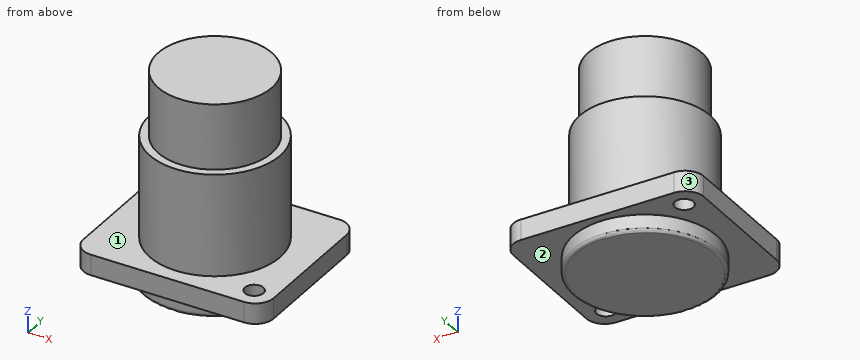
from build123d import *

# Parameters (mm, degrees)
SZKIC1_R                    = 11.6
DODANIE_WYCI_GNI_CIE1_DEPTH = 2.7
ZAOKR_GLENIE1_R             = 0.5
SZKIC2_W                    = 30.8
SZKIC2_H                    = 25.8
DODANIE_WYCI_GNI_CIE2_DEPTH = 3.33
SZKIC3_R                    = 10.55
DODANIE_WYCI_GNI_CIE3_DEPTH = 16.5
SZKIC4_R                    = 9.2
DODANIE_WYCI_GNI_CIE4_DEPTH = 10.6
SZKIC5_R                    = 1.5
WYTNIJ_WYCI_GNI_CIE1_DEPTH  = 10.6
ZAOKR_GLENIE2_R             = 3


with BuildPart() as part:
    # Szkic1 → Dodanie-wyciągnięcie1 (new body)
    with BuildSketch(Plane.XY):
        with Locations(Location((0, 0, 0), (0, 0, 180))):
            Circle(SZKIC1_R)
    extrude(amount=DODANIE_WYCI_GNI_CIE1_DEPTH)

    # Zaokrąglenie1
    zaokr_glenie1_edges = [part.edges().sort_by_distance(p)[0] for p in [
        (11.6, 0, 0),
    ]]
    fillet(zaokr_glenie1_edges, radius=ZAOKR_GLENIE1_R)

    # Szkic2 → Dodanie-wyciągnięcie2 (add)
    with BuildSketch(Plane.XY.offset(2.7)):
        Rectangle(SZKIC2_W, SZKIC2_H)
    extrude(amount=DODANIE_WYCI_GNI_CIE2_DEPTH)

    # Szkic3 → Dodanie-wyciągnięcie3 (add)
    with BuildSketch(Plane.XY.offset(6.03)):
        Circle(SZKIC3_R)
    extrude(amount=DODANIE_WYCI_GNI_CIE3_DEPTH)

    # Szkic4 → Dodanie-wyciągnięcie4 (add)
    with BuildSketch(Plane.XY.offset(22.53)):
        Circle(SZKIC4_R)
    extrude(amount=DODANIE_WYCI_GNI_CIE4_DEPTH)

    # Szkic5 → Wytnij-wyciągnięcie1 (cut)
    with BuildSketch(Plane(origin=(0, 0, 2.7), x_dir=(-1, 0, 0), z_dir=(0, 0, -1))):
        with Locations((-12, -9.5)):
            Circle(SZKIC5_R)
        with Locations((12, 9.5)):
            Circle(SZKIC5_R)
    extrude(amount=-WYTNIJ_WYCI_GNI_CIE1_DEPTH, mode=Mode.SUBTRACT)

    # Zaokrąglenie2
    zaokr_glenie2_edges = [part.edges().sort_by_distance(p)[0] for p in [
        (-15.4, 12.9, 4.365),
        (-15.4, -12.9, 4.365),
        (15.4, -12.9, 4.365),
        (15.4, 12.9, 4.365),
    ]]
    fillet(zaokr_glenie2_edges, radius=ZAOKR_GLENIE2_R)


solid = part.part
Read the model definition and answer for the solid it produces. Units are mm, in the model's axes. Face numbers are marked on the shaded views. A direction names the side the tool comes from. Coordinates: 2 decimals unless noted, no trailing zeros. Loops run counter-clockwise (first coordinate to the right, second up) from the corner with the lowest first, then second, coordinate; pieces in that order, holes last. Notation, with made-up numbers: (-26, 55) -> (-10, 55) arc R20 ccw to (-10, 77) -> close; hole circle Ø7 at (63.5, -9). An arc over 180 degrees is marked (long way). Write item = value, one per line. Start each with the question number.
1) The part is cut by section C-C, the plane y = 0. Determine the outline of the cut face in (x, z), plus the area to 3 significant figures.
2) For the marked faces 1, 2 and 3, determine the directions among +Z, -Z, +X, -X, +Y, -Y from which every point of the face is accessible in a straight line to the end or side of a thin tool.
3) The part is cut by section B-B, the plane x = 0. Determine the outline of the cut face in (y, z).
4) The part is cut by section A-A, the plane z = 4. Determine the outline of the cut face in (x, y).
5) The part is cut by section D-D, the plane z = 20. Determine the outline of the cut face in (x, y), plus the area to 3 significant figures.
6) Find the intervals of material crossed by L1, parallel to Y at x = 12, z = 4; L2, parallel to Y at x = -12, z = 5.05; L3, parallel to Z at x = -8, y = 7, in increasing order. Write a range as from..to.
7) Given P1, Ø8, axis at x = 0, y = -4.5, coming from the -Z side; P2, Ø3, axis at x = 8.5, z = 23, coming from the -Y side; P3, Ø8, axis at y = -7.5, z = 29.5, coming from the +X side; P4, Ø3, axis at y = 0.5, z = 21, coming from the -X side, each flat-ended and moving along its own axis, determine where each tip first touches the part or whether it passes through.
Result:
q1.outline = (-15.4, 2.7) -> (-11.6, 2.7) -> (-11.6, 0.5) arc R0.5 ccw to (-11.1, 0) -> (11.1, 0) arc R0.5 ccw to (11.6, 0.5) -> (11.6, 2.7) -> (15.4, 2.7) -> (15.4, 6.03) -> (10.55, 6.03) -> (10.55, 22.53) -> (9.2, 22.53) -> (9.2, 33.13) -> (-9.2, 33.13) -> (-9.2, 22.53) -> (-10.55, 22.53) -> (-10.55, 6.03) -> (-15.4, 6.03) -> close
q1.area = 708 mm²
q2.face_1 = +Z
q2.face_2 = -Z
q2.face_3 = +Z, -Z, -X, +Y
q3.outline = (-12.9, 2.7) -> (-11.6, 2.7) -> (-11.6, 0.5) arc R0.5 ccw to (-11.1, 0) -> (11.1, 0) arc R0.5 ccw to (11.6, 0.5) -> (11.6, 2.7) -> (12.9, 2.7) -> (12.9, 6.03) -> (10.55, 6.03) -> (10.55, 22.53) -> (9.2, 22.53) -> (9.2, 33.13) -> (-9.2, 33.13) -> (-9.2, 22.53) -> (-10.55, 22.53) -> (-10.55, 6.03) -> (-12.9, 6.03) -> close
q4.outline = (-15.4, -9.9) arc R3 ccw to (-12.4, -12.9) -> (12.4, -12.9) arc R3 ccw to (15.4, -9.9) -> (15.4, 9.9) arc R3 ccw to (12.4, 12.9) -> (-12.4, 12.9) arc R3 ccw to (-15.4, 9.9) -> close; hole circle Ø3 at (-12, 9.5); hole circle Ø3 at (12, -9.5)
q5.outline = circle Ø21.1 at (0, 0)
q5.area = 350 mm²
q6.L1 = -12.9..-11, -8..12.9
q6.L2 = -12.9..8, 11..12.9
q6.L3 = 0..6.03
q7.P1 = 0
q7.P2 = -7.83
q7.P3 = 8.51
q7.P4 = -10.55
